Input: part model. Units: mm. Frame: model coordinates. Face numbers are marked on the shaded views. A direction names the side the tool comes from. Coordinates: 2 decimals unless noted, no trailing zeros. Order: outer loops, then holes, each group sorted by start corner. A loop starts at its lowest first (then second) coordinate and runs counter-clockwise, first axis right, second up.
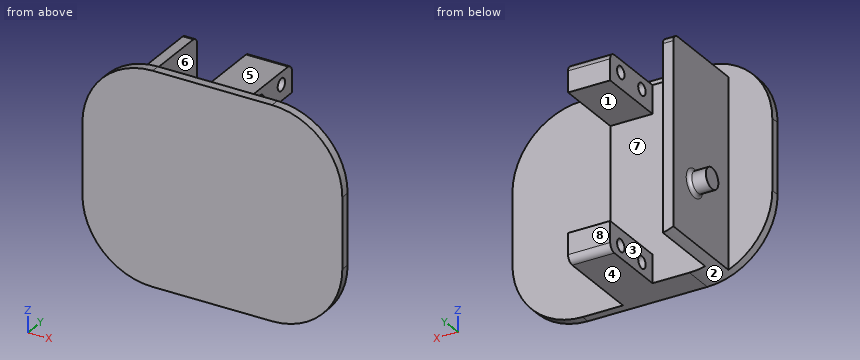
from build123d import *

# Parameters (mm, degrees)
ESQUISSE1_W             = 74
ESQUISSE1_H             = 60
BOSS_EXTRU_1_DEPTH      = 2.5
ESQUISSE2_W             = 30
ESQUISSE2_H             = 55
BOSS_EXTRU_2_DEPTH      = 6
ESQUISSE4_W             = 12
ESQUISSE4_H             = 8
BOSS_EXTRU_3_DEPTH      = 20
ESQUISSE5_R             = 1.75
ENL_V_MAT_EXTRU_1_DEPTH = 20
ESQUISSE6_R             = 2.95
BOSS_EXTRU_4_DEPTH      = 5
CONG_1_R                = 1
CONG_2_R                = 20
CONG_3_R                = 2


with BuildPart() as part:
    # Esquisse1 → Boss.-Extru.1 (new body)
    with BuildSketch(Plane(origin=(0, 0, 0), x_dir=(1, 0, 0), z_dir=(0, 1, 0))):
        with Locations((37, 30)):
            Rectangle(ESQUISSE1_W, ESQUISSE1_H)
    extrude(amount=BOSS_EXTRU_1_DEPTH)

    # Esquisse2 → Boss.-Extru.2 (add)
    with BuildSketch(Plane(origin=(0, 2.5, 0), x_dir=(1, 0, 0), z_dir=(0, 1, 0))):
        with Locations((27.5, 32.5)):
            Rectangle(ESQUISSE2_W, ESQUISSE2_H)
    extrude(amount=BOSS_EXTRU_2_DEPTH)

    # Esquisse4 → Boss.-Extru.3 (add)
    with BuildSketch(Plane(origin=(0, 8.5, 0), x_dir=(1, 0, 0), z_dir=(0, 1, 0))):
        with Locations((36.5, 56)):
            Rectangle(ESQUISSE4_W, ESQUISSE4_H)
        Polygon((12.5, 60), (12.5, 52), (12.5, 13), (12.5, 5), (15.5, 5), (15.5, 13), (15.5, 52), (15.5, 60), align=None)
        with Locations((36.5, 9)):
            Rectangle(ESQUISSE4_W, ESQUISSE4_H)
    extrude(amount=BOSS_EXTRU_3_DEPTH)

    # Esquisse5 → Enlèv. mat.-Extru.1 (cut)
    with BuildSketch(Plane(origin=(42.5, 0, 0), x_dir=(0, 0, -1), z_dir=(1, 0, 0))):
        with Locations((8.5, 23.5)):
            Circle(ESQUISSE5_R)
        with Locations((8.5, 13.5)):
            Circle(ESQUISSE5_R)
        with Locations((56.5, 23.5)):
            Circle(ESQUISSE5_R)
        with Locations((56.5, 13.5)):
            Circle(ESQUISSE5_R)
    extrude(amount=-ENL_V_MAT_EXTRU_1_DEPTH, mode=Mode.SUBTRACT)

    # Esquisse6 → Boss.-Extru.4 (add)
    with BuildSketch(Plane.ZY.offset(-12.5)):
        with Locations((-42, 18.5)):
            Circle(ESQUISSE6_R)
    extrude(amount=BOSS_EXTRU_4_DEPTH)

    # Congé1
    cong_1_edges = [part.edges().sort_by_distance(p)[0] for p in [
        (12.5, 18.5, -44.95),
    ]]
    fillet(cong_1_edges, radius=CONG_1_R)

    # Congé2
    cong_2_edges = [part.edges().sort_by_distance(p)[0] for p in [
        (74, 1.25, -60),
        (74, 1.25, 0),
        (0, 1.25, 0),
        (0, 1.25, -60),
    ]]
    fillet(cong_2_edges, radius=CONG_2_R)

    # Congé3
    cong_3_edges = [part.edges().sort_by_distance(p)[0] for p in [
        (36.5, 28.5, -60),
        (14, 28.5, -5),
        (36.5, 28.5, -5),
    ]]
    fillet(cong_3_edges, radius=CONG_3_R)


solid = part.part
Item 1: Cut plane C-C on z = -24. Return loops of the section in (x, y).
Response values:
outline: (0, 0) - (74, 0) - (74, 2.5) - (42.5, 2.5) - (42.5, 8.5) - (15.5, 8.5) - (15.5, 28.5) - (12.5, 28.5) - (12.5, 2.5) - (0, 2.5) - close
Item 2: Ray query, probe 1 along Y at (x, z) = (40.25, -56.5); probe 2 along Z at (x, y) = (40.5, 11.5); probe 3 along X at (y, z) = (15, -21). Return the intervals inside material, ascending.
Response values:
probe 1: y = 0 to 11.75, 15.25 to 21.75, 25.25 to 28.5
probe 2: z = -60 to -52, -13 to -5
probe 3: x = 12.5 to 15.5
Item 3: Cut plane A-A on y = 18.5. Return loops of the section in (x, z).
Response values:
outline: (7.5, -44.95) - (11.5, -44.95) arc R1 cw to (12.5, -45.95) - (12.5, -58.54) arc R20 ccw to (15.5, -59.49) - (15.5, -5) - (12.5, -5) - (12.5, -38.05) arc R1 cw to (11.5, -39.05) - (7.5, -39.05) - close; (30.5, -60) - (42.5, -60) - (42.5, -52) - (30.5, -52) - close; (30.5, -13) - (42.5, -13) - (42.5, -5) - (30.5, -5) - close
Item 4: Pin query (flat end, axial travel): pin 1 Ø13 at (x, y) = (37.5, 23) entering from +Z; pin 2 Ø8 at (y, z) = (13, -33) entering from -X; pin 3 Ø5.5 at (y, z) = (13.5, -56.5) entering from +X; pin 4 Ø1.5 at (x, y) = (11, 14) entering from +Z. Return the tip coordinate at first contact, or that it passes through.
Response values:
pin 1: stops at z = -5
pin 2: stops at x = 12.5
pin 3: stops at x = 42.5
pin 4: passes through
Item 5: Cut plane B-B on y = 13.5. Return loops of the section in (x, z).
Response values:
outline: (12.5, -58.54) arc R20 ccw to (15.5, -59.49) - (15.5, -5) - (12.5, -5) - close; (30.5, -60) - (42.5, -60) - (42.5, -58.25) - (30.5, -58.25) - close; (30.5, -54.75) - (42.5, -54.75) - (42.5, -52) - (30.5, -52) - close; (30.5, -13) - (42.5, -13) - (42.5, -10.25) - (30.5, -10.25) - close; (30.5, -6.75) - (42.5, -6.75) - (42.5, -5) - (30.5, -5) - close
Item 6: Cut plane D-D on z = -56.5. Return loops of the section in (x, y).
Response values:
outline: (8.7, 0) - (65.3, 0) - (65.3, 2.5) - (42.5, 2.5) - (42.5, 11.75) - (30.5, 11.75) - (30.5, 8.5) - (15.5, 8.5) - (15.5, 28.5) - (12.5, 28.5) - (12.5, 2.5) - (8.7, 2.5) - close; (30.5, 15.25) - (42.5, 15.25) - (42.5, 21.75) - (30.5, 21.75) - close; (30.5, 25.25) - (42.5, 25.25) - (42.5, 28.5) - (30.5, 28.5) - close
Item 7: Access query for the marked faces 4, 5, 6, 7 and 8. Directions: +Z, -Z, +X, -X, +Y, -Y. A direction counts if a zero-diameter tool reaches every point of the face in a straight line with its end or side. Return the directions, or none.
Response values:
face 4: -Z, +X, -X, +Y, -Y
face 5: +Z, +X, -X, +Y
face 6: +Z, -Z, +Y
face 7: +Y
face 8: +Z, -Z, +X, -X, +Y
Item 8: Draft query along X for the marked faces 1, 2 and 3. Return one class per face: pulls with the +X half, pulls with the -X half, needs draft (parallel to the pull), parting line crosses it, or undercut.
Response values:
face 1: needs draft
face 2: pulls with the -X half
face 3: undercut
